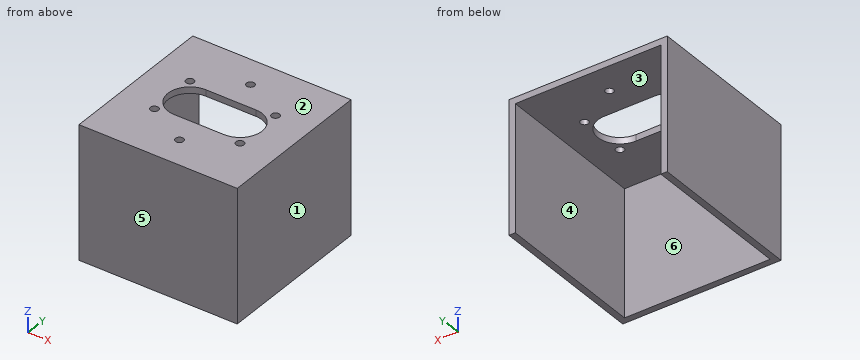
Autodesk Inventor part; units mm, degrees
ref_plane "YZ Plane" through (0, 0, 0) normal (1, 0, 0) x (0, 1, 0)
ref_plane "XZ Plane" through (0, 0, 0) normal (0, 1, 0) x (-1, 0, 0)
ref_plane "XY Plane" through (0, 0, 0) normal (0, 0, 1) x (1, 0, 0)
sketch "Sketch1" plane through (0, 0, 0) normal (0, 0, 1) x (1, 0, 0)
  circle A0 centre (0, 0) radius 18.38
  circle A1 centre (13.5143, 7.8025) radius 1.255
  circle A2 centre (0, 15.605) radius 1.255
  circle A3 centre (-13.5143, 7.8025) radius 1.255
  circle A4 centre (-13.5143, -7.8025) radius 1.255
  circle A5 centre (0, -15.605) radius 1.255
  circle A6 centre (13.5143, -7.8025) radius 1.255
  circle A7 centre (7.9, 0) radius 5.98
  line L0 (25, 25) -> (-25, 25)
  line L1 (-25, 25) -> (-25, -25)
  line L2 (-25, -25) -> (25, -25)
  line L3 (25, -25) -> (25, 25)
  line L4 (25, 25) -> (-25, -25) construction
  line L5 (-25, 25) -> (25, -25) construction
  circle A8 centre (7.9, 0) radius 6.98
  line L6 (7.9, -6.98) -> (-7.9, -6.98)
  line L7 (7.9, 6.98) -> (-7.9, 6.98)
  circle A9 centre (-7.9, 0) radius 6.98
  line L8 (23, 23) -> (-23, 23)
  line L9 (-23, 23) -> (-23, -23)
  line L10 (-23, -23) -> (23, -23)
  line L11 (23, -23) -> (23, 23)
  line L12 (-23, 23) -> (-23, 25)
  line L13 (23, 23) -> (23, 25)
  line L14 (23, -23) -> (23, -25)
  point P0 (0, 0)
  dimension "d0" = 50
  dimension "d1" = 50
  dimension "d2" = 1
  dimension "d3" = 15.8
  dimension "d6" = 2
extrude "Extrusion1" add sketch "Sketch1" along normal blind 2 contours A0 | L3 L2 L14 L11 L13 L0 | L13 L8 L12 L0 | L12 L9 L10 L14 L2 L1 L0 | L11 L10 L9 L8
extrude "Extrusion2" add sketch "Sketch1" against normal blind 40 contours L3 L2 L14 L11 L13 L0 | L12 L9 L10 L14 L2 L1 L0
thread "Thread1"
thread "Thread2"
thread "Thread3"
thread "Thread4"
thread "Thread5"
thread "Thread6"
properties part number "drivemotorcasing"
Geometry check sheet. Reference: the model listing, model coordinates, mm. Face numbers are marked on the shaded views. A direction names the side the tool comes from. Coordinates: 2 decimals unless noted, no trailing zeros. Loops run counter-clockwise (first coordinate to the right, second up) from the corner with the lowest first, then second, coordinate; pieces in that order, holes last. Notation, with made-up numbers: (-15, 81) -> (44, 81) arc R28 cw to (44, 108) -> close; hole circle Ø3 at (57.25, 86.25). An arc over 180 degrees is marked (long way). Put each result on its own line as item: value.
1) Cross-section at A-A on x = 2. Record the boundary of the cut face in (y, z), plus the area to 3 significant figures.
Result set:
outline: (-25, -40) -> (-23, -40) -> (-23, 0) -> (-6.98, 0) -> (-6.98, 2) -> (-25, 2) -> close; (6.98, 0) -> (25, 0) -> (25, 2) -> (6.98, 2) -> close
area: 152 mm^2
2) Cross-section at C-C on x = 14. Record the boundary of the cut face in (y, z), plus the area to 3 significant figures.
Result set:
outline: (-25, -40) -> (-23, -40) -> (-23, 0) -> (-8.96, 0) -> (-8.96, 2) -> (-25, 2) -> close; (-6.65, 0) -> (-3.39, 0) -> (-3.39, 2) -> (-6.65, 2) -> close; (3.39, 0) -> (6.65, 0) -> (6.65, 2) -> (3.39, 2) -> close; (8.96, 0) -> (25, 0) -> (25, 2) -> (8.96, 2) -> close
area: 157 mm^2
3) Cross-section at B-B on y = 0. Record the boundary of the cut face in (x, z), plus the area to 3 significant figures.
Result set:
outline: (-25, -40) -> (-23, -40) -> (-23, 0) -> (-14.88, 0) -> (-14.88, 2) -> (-25, 2) -> close; (14.88, 0) -> (23, 0) -> (23, -40) -> (25, -40) -> (25, 2) -> (14.88, 2) -> close
area: 200 mm^2
4) Gauge pin test, flat ends, axial feed: pin 1 Ø6 at (x, y) = (18.5, -9.5) entering from -Z; pin 2 Ø3 at (x, z) = (-7.5, -5.5) entering from +Y; pin 3 Ø4 at (x, y) = (0, 15.605) entering from +Z. Record the tip position at first contact, or that the pin passes through.
Result set:
pin 1: stops at z = 0
pin 2: stops at y = -23
pin 3: stops at z = 2
5) Tool access check on the marked faces 5 and 6. Record the directions out of +Z, -Z, +X, -X, +Y, -Y that give a thin tool (end or side, any length) a straight path to the whole face; none if there is none.
Result set:
face 5: +Z, -Z, +X, -X, -Y
face 6: -Z, +Y
6) Release check for a two-part mould opening along X. For the marked faces 1, 2, 3 and 4 record: released by +X, released by -X, zero draft, split by the parting line, or undercut.
Result set:
face 1: released by +X
face 2: zero draft
face 3: undercut
face 4: undercut
7) Thickness scan on line 1 (Y direction, x = 0, z = 1.35); line 2 (X direction, y = -18.5, z = -15); line 3 (Z direction, x = 9, y = -15). Record the ranges inside material, lowest first.
Result set:
line 1: y = -25 to -16.86, -14.35 to -6.98, 6.98 to 14.35, 16.86 to 25
line 2: x = -25 to -23, 23 to 25
line 3: z = 0 to 2
8) Cross-section at D-D on z = -21. Record the boundary of the cut face in (x, y), plus the area to 3 significant figures.
Result set:
outline: (-25, -25) -> (25, -25) -> (25, 25) -> (23, 25) -> (23, -23) -> (-23, -23) -> (-23, 25) -> (-25, 25) -> close
area: 292 mm^2
